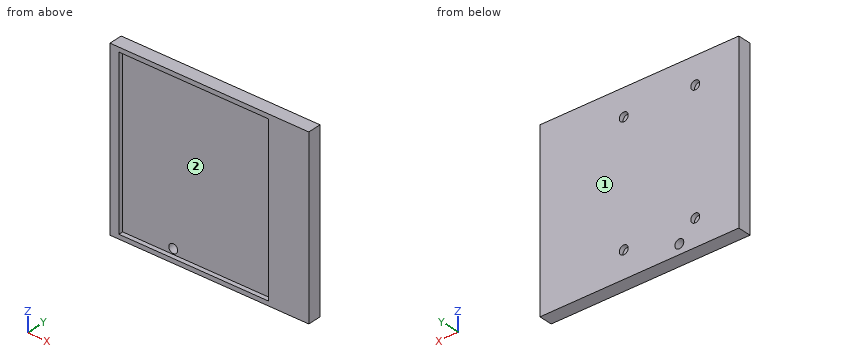
from build123d import *

# Parameters (mm, degrees)
SKETCH1_W               = 355.26
SKETCH1_H               = 390
BOSS_EXTRUDE1_DEPTH     = 30
SKETCH3_W               = 390
SKETCH3_H               = 30
BOSS_EXTRUDE2_DEPTH     = 90
SKETCH4_R               = 10
CUT_EXTRUDE1_DEPTH      = 10
MIRROR2_COPY_1_SKETCH_R = 10
MIRROR2_COPY_1_DEPTH    = 10
SKETCH7_W               = 335.26
SKETCH7_H               = 370
CUT_EXTRUDE3_DEPTH      = 10
SKETCH8_R               = 10
CUT_EXTRUDE4_DEPTH      = 87


with BuildPart() as part:
    # Sketch1 → Boss-Extrude1 (new body)
    with BuildSketch(Plane(origin=(0, 0, 0), x_dir=(1, 0, 0), z_dir=(0, 1, 0))):
        with Locations((177.63, -195)):
            Rectangle(SKETCH1_W, SKETCH1_H)
    extrude(amount=BOSS_EXTRUDE1_DEPTH)

    # Sketch3 → Boss-Extrude2 (add)
    with BuildSketch(Plane(origin=(355.26, 0, 0), x_dir=(0, 0, -1), z_dir=(1, 0, 0))):
        with Locations((-195, 15)):
            Rectangle(SKETCH3_W, SKETCH3_H)
    extrude(amount=BOSS_EXTRUDE2_DEPTH)

    # Sketch4 → Cut-Extrude1 (cut)
    with BuildSketch(Plane(origin=(0, 30, 0), x_dir=(1, 0, 0), z_dir=(0, 1, 0))):
        with Locations(Location((97.63, -60, 0), (0, 0, 270))):
            Circle(SKETCH4_R)
    cut_extrude1 = extrude(amount=-CUT_EXTRUDE1_DEPTH, mode=Mode.SUBTRACT)

    # Mirror1: Cut-Extrude1 across plane
    add(cut_extrude1.mirror(Plane.ZY.offset(-177.63)), mode=Mode.SUBTRACT)

    # Mirror2: Cut-Extrude1 across plane
    add(cut_extrude1.mirror(Plane.XY.offset(195)), mode=Mode.SUBTRACT)

    # Mirror2 copy 1 sketch → Mirror2 copy 1 (cut)
    with BuildSketch(Plane(origin=(355.26, 30, 390), x_dir=(-1, 0, 0), z_dir=(0, 1, 0))):
        with Locations(Location((97.63, -60, 0), (0, 0, 270))):
            Circle(MIRROR2_COPY_1_SKETCH_R)
    extrude(amount=-MIRROR2_COPY_1_DEPTH, mode=Mode.SUBTRACT)

    # Sketch7 → Cut-Extrude3 (cut)
    with BuildSketch(Plane.XZ):
        with Locations((187.63, 195)):
            Rectangle(SKETCH7_W, SKETCH7_H)
    extrude(amount=-CUT_EXTRUDE3_DEPTH, mode=Mode.SUBTRACT)

    # Sketch8 → Cut-Extrude4 (cut)
    with BuildSketch(Plane(origin=(0, 30, 0), x_dir=(1, 0, 0), z_dir=(0, 1, 0))):
        with Locations(Location((133.244825989, -21.940410103, 0), (0, 0, 270))):
            Circle(SKETCH8_R)
    extrude(amount=-CUT_EXTRUDE4_DEPTH, mode=Mode.SUBTRACT)


solid = part.part
Source: CAD feature listing. Evaluate the final solid. Frame: model axes, mm. Face numbers are marked on the shaded views. Coordinates: 2 decimals unless noted, no trailing zeros. Order: outer loops, then holes, each group sorted by start corner. A loop starts at its lowest first (then second) coordinate and runs counter-clockwise, first axis right, second up.
Item 1: Pull-direction query (X, two-part tool) for the marked faces 1 and 2; classes: pulls with the +X half, pulls with the -X half, needs draft (parallel to the pull), parting line crosses it, or undercut.
Output values:
face 1: needs draft
face 2: undercut
Item 2: Cut plane C-C (z = 157). Return loops of the section in (x, y).
Output values:
outline: (0, 0) - (20, 0) - (20, 10) - (355.26, 10) - (355.26, 0) - (445.26, 0) - (445.26, 30) - (0, 30) - close
Item 3: First-contact query: P1, Ø10, axis at x = 292, z = 112, coming from the -Y side; P2, Ø10, axis at x = 102.5, z = 325.5, coming from the +Y side; P3, Ø12, axis at x = 257.63, z = 330, coming from the +Y side. Flat tips, straight axial feed; report the tip coordinate or a pass-through.
Output values:
P1: stops at y = 10
P2: stops at y = 30
P3: stops at y = 20
Item 4: Material intervals for line 1 (X direction, y = 23, z = 60); line 2 (Z direction, x = 257.63, y = 23); line 3 (X direction, y = 6.25, z = 96), sorted ascending.
Output values:
line 1: x = 0 to 87.63, 107.63 to 247.63, 267.63 to 445.26
line 2: z = 0 to 50, 70 to 320, 340 to 390
line 3: x = 0 to 20, 355.26 to 445.26
Item 5: Cut plane B-B (x = 284.5). Return loops of the section in (y, z).
Output values:
outline: (0, 0) - (30, 0) - (30, 390) - (0, 390) - (0, 380) - (10, 380) - (10, 10) - (0, 10) - close
Item 6: Cut plane A-A (z = 60). Return loops of the section in (x, y).
Output values:
outline: (0, 0) - (20, 0) - (20, 10) - (355.26, 10) - (355.26, 0) - (445.26, 0) - (445.26, 30) - (267.63, 30) - (267.63, 20) - (247.63, 20) - (247.63, 30) - (107.63, 30) - (107.63, 20) - (87.63, 20) - (87.63, 30) - (0, 30) - close
